Here's the drawing with two shaded views (mm, measured from the low corner). I have some questions. Round coordinates to 2 decimals unless told otherwise and drop trailing zeros. Write each loop counter-clockwise with the first axis right and the second up, starting at its lowest first coordinate (ties: lowest second). Pieces come first, ordered by that corner, then holes. Notation, with made-up numbers: (78, 64.5) -> (134, 64.5) arc R19 cw to (134, 99.5) -> close; hole circle Ø7 at (30.5, 65). An arc over 180 degrees is marked (long way). Use CSV: the item, a comma, the result in double quotes.
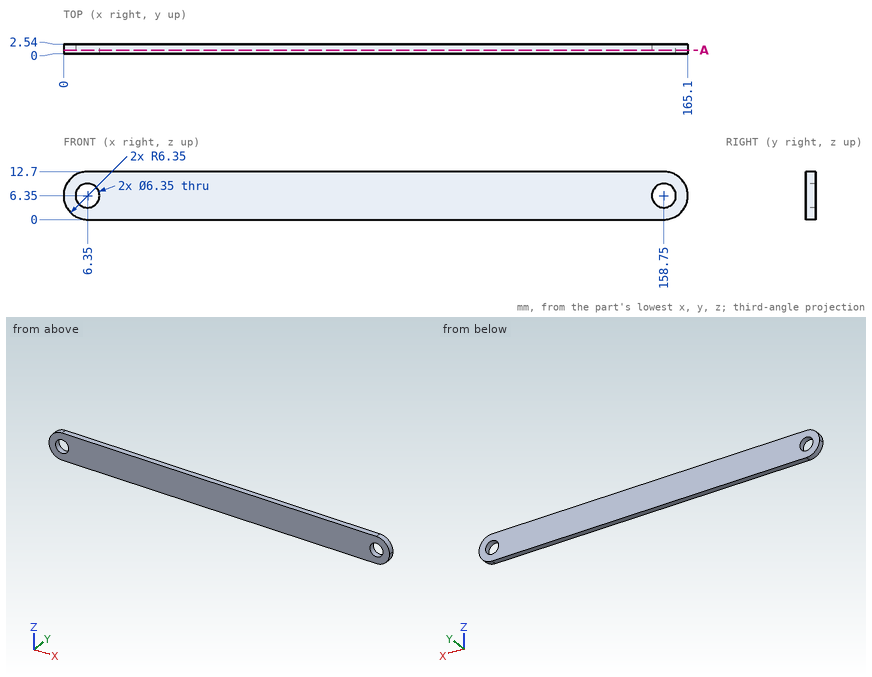
Q1. Suppose I cut it at A-A (y = 0.9). Write out the boundary of the cut face in (x, z) (3 decimals), and give its area (3 significant figures).
Resolved:
outline,"(6.35, 0) -> (158.75, 0) arc R6.35 ccw to (158.75, 12.7) -> (6.35, 12.7) arc R6.35 ccw to start; hole circle Ø6.35 at (6.35, 6.35); hole circle Ø6.35 at (158.75, 6.35)"
area,"2,000 mm^2"
Q2. Please list where these lines run through material, in increasing order: probe 1 along Z at (x, y) = (158.75, 1.5) (3 decimals); probe 2 along X at (y, z) = (1.35, 7.75); probe 3 along Z at (x, y) = (8, 1.95).
Resolved:
probe 1,"z = 0 to 3.175, 9.525 to 12.7"
probe 2,"x = 0.16 to 3.5, 9.2 to 155.9, 161.6 to 164.94"
probe 3,"z = 0 to 3.64, 9.06 to 12.7"
Q3. Will this pin go through, and if not, where does the flat tip stop? P1, Ø1, axis at y = 0.5, z = 7, coming from the -X side.
Resolved:
P1,"stops at x = 0"
